Autodesk Inventor part; units mm, degrees
ref_plane "YZ Plane" through (0, 0, 0) normal (1, 0, 0) x (0, 1, 0)
ref_plane "XZ Plane" through (0, 0, 0) normal (0, 1, 0) x (-1, 0, 0)
ref_plane "XY Plane" through (0, 0, 0) normal (0, 0, 1) x (1, 0, 0)
sketch "Skizze1" plane through (0, 0, 0) normal (1, 0, 0) x (0, 1, 0)
  line L0 (-35, 0) -> (35, 0) construction
  line L1 (0, 42) -> (0, -42) construction
  line L2 (-25, -30) -> (25, -30)
  line L3 (25, -30) -> (25, 30)
  line L4 (25, 30) -> (-25, 30)
  line L5 (-25, 30) -> (-25, -30)
  line L6 (-25, -30) -> (25, 30) construction
  line L7 (25, -30) -> (-25, 30) construction
  point P0 (0, 0)
  dimension "d0" = 50
  dimension "d1" = 60
extrude "Grundkörper" add sketch "Skizze1" along normal mid plane 30
sketch "Skizze2" plane through (15, 0, 0) normal (1, 0, 0) x (0, 0, -1)
  line L0 (-30, 25) -> (-30, -25) construction
  line L1 (0, -35) -> (0, 35) construction
  line L2 (-42, 0) -> (42, 0) construction
  line L3 (-30, -15) -> (10, -15)
  line L4 (10, -15) -> (10, 15)
  line L5 (10, 15) -> (-30, 15)
  line L6 (-30, 15) -> (-30, -15)
  line L7 (30, -25) -> (30, 25) construction
  line L8 (30, -8.4) -> (25, -8.4)
  line L9 (17, -0.4) -> (17, 0.4)
  line L10 (25, 8.4) -> (30, 8.4)
  line L11 (30, -8.4) -> (30, 8.4)
  arc A0 (17, -0.4) -> (25, -8.4) centre (25, -0.4) ccw
  arc A1 (25, 8.4) -> (17, 0.4) centre (25, 0.4) ccw
  point P0 (0, 0)
  dimension "d4" = 40
  dimension "d5" = 30
  dimension "d14" = 13
  dimension "d15" = 16.8
  dimension "d16" = 8
extrude "Ausschnitt" cut sketch "Skizze2" against normal through all
sketch "Skizze4" plane through (-15, -25, -30) normal (0, -1, 0) x (1, 0, 0)
  line L0 (30, 20) -> (0, 20) construction
  line L1 (30, 60) -> (0, 60) construction
  line L2 (15, 72) -> (15, -12)
  line L3 (0, 40) -> (30, 40) construction
  line L4 (0, 0) -> (0, 60) construction
  line L5 (30, 60) -> (30, 0) construction
  point P0 (15, 30)
  point P1 (15, 50)
  point P2 (15, 30)
  dimension "d19" = 40
  dimension "d20" = 20
  dimension "d21" = 20
hole "DIN7984_M8_Boh" at (0, -25, 20) at (0, -25, 0) direction (0, 1, 0) diameter 9 end up to surface counterbore diameter 15 counterbore depth 5.4
mirror "Spiegeln_DIN7984_M8_Boh" about plane through (0, 0, 0) normal (0, 1, 0) of "DIN7984_M8_Boh"
sketch "Skizze5" plane through (15, -25, -30) normal (0, 0, -1) x (-1, 0, 0)
  line L0 (0, 0) -> (30, 0) construction
  line L1 (30, 16.6) -> (0, 16.6) construction
  line L2 (30, 50) -> (0, 50) construction
  line L3 (0, 33.4) -> (30, 33.4) construction
  line L4 (15, -10) -> (15, 60) construction
  line L5 (-6, 25) -> (36, 25) construction
  line L6 (15, 16.6) -> (15, 0) construction
  point P0 (15, 25)
  point P1 (15, 8.3)
  point P2 (15, 41.7)
  dimension "d29" = 33.4
hole "M5x10" at (0, -16.7, -30) at (0, 16.7, -30) direction (0, 0, 1) diameter 4.134 depth 14.2 tip angle 118 countersink diameter 5 countersink angle 90
sketch "Skizze" plane through (15, -25, -30) normal (0, 0, -1) x (-1, 0, 0)
  circle A0 centre (15, 8.3) radius 2.5
  line L0 (30, 16.6) -> (0, 16.6)
  line L1 (0, 0) -> (0, 16.6)
  line L2 (0, 0) -> (30, 0)
  line L3 (30, 16.6) -> (30, 0)
  circle A1 centre (15, 41.7) radius 2.5
  line L4 (0, 33.4) -> (30, 33.4)
  line L5 (30, 50) -> (30, 33.4)
  line L6 (30, 50) -> (0, 50)
  line L7 (0, 33.4) -> (0, 50)
  line L8 (0, 16.6) -> (0, 24.6)
  line L9 (0, 24.6) -> (0, 25.4)
  line L10 (0, 25.4) -> (0, 33.4)
  line L11 (30, 33.4) -> (30, 25.4)
  line L12 (30, 25.4) -> (30, 24.6)
  line L13 (30, 24.6) -> (30, 16.6)
  point P0 (15, 25)
chamfer "Fase_Allgemein" distance 4 angle 45 4 edges at (15, -25, 0) (-15, -25, 0) (15, 25, 0) (-15, 25, 0)
chamfer "Fase" distance 0.5 angle 45 15 edges at (15, -6.0569, -19.3431) (15, 0, -17) (15, 6.0569, -19.3431) (15, 8.4, -27.5) (15, -8.4, -27.5) (-15, 6.0569, -19.3431) (-15, 0, -17) (-15, -6.0569, -19.3431) (-15, -8.4, -27.5) (-15, 8.4, -27.5) (-15, 0, -10) (-15, 15, 10) (15, -15, 10) (15, 0, -10) (15, 15, 10)
equation "\"d20\" = 0.5 * d19"
properties part number "200-50-WHEEL-CONNECTOR-30MM-01" material "Aluminium 6061"
The listing builds one solid part. Answer for the finished solid, in the listing's coordinates (mm). A direction names the side the tool comes from. Round coordinates to 2 decimals unless told otherwise and drop trailing zeros. Order: outer loops, then holes, each group sorted by start corner. A loop starts at its lowest first (then second) coordinate and runs counter-clockwise, first axis right, second up. Notation, with made-up numbers: (22, 59) -> (36, 59) arc R18 cw to (36, 67) -> close; hole circle Ø4 at (15, 84.25). An arc over 180 degrees is marked (long way). Answer as CSV lines item,"result". Start each with the question number.
(1) A tool of negligible diameter and unlimited length cuts with its end or side. For faces 5 (the face through (0, 19.6, 25)), 6 (the face through (0, -19.6, 15)), 7 (the face through (0.203, 6.119, -19.406)), 8 (the face through (0, -15, 10)), from which of +Z, -Z, +X, -X, +Y, -Y can it reach the whole face along a straight path? Write none if from no direction.
(2) Flat-ended cylindrical pins translate along their axes: pin 1 Ø11.5 at (x, z) = (0, 0) entering from +Y; pin 2 Ø9 at (x, z) = (-6, 3.5) entering from +Y; pin 3 Ø2 at (x, y) = (-0.5, 13.5) entering from +Z; pin 4 Ø0.9 at (x, y) = (-7, 0) entering from -Z. Find the tip coordinate at first contact, or state that the pin passes through.
(3) For a pull along X with two mould halves and no side action, classify faces 1 (the face through (14.64, 6.22, -19.31)), 2 (the face through (-4.46, -17.27, 0.59)), 3 (the face through (-13, -23, 0)), 4 (the face through (0, -20, 30)) as +X half, -X half, draft (parallel to the pull), parting line (faces both ways), or undercut.
(4) The part is cut by section C-C (x = -10). Determine the outline of the cut face in (y, z).
(5) Find the intervals of material crossed by probe 1 along Y at (x, z) = (0, -27); probe 2 along Y at (x, z) = (-2, 5.5); probe 3 along Z at (x, y) = (0, 21), in increasing order. Write a range as from..to.
(6) The part is cut by section A-A (z = 20). Count the separate pieces of the cut face and the enclosed holes in it, then the cut area to 3 significant figures.
(7) The part is cut by section B-B (z = 10.5). Determine the outline of the cut face in (x, y), then the cut area to 3 significant figures.
Evaluation:
1,face 5,"+Y"
1,face 6,"-Y"
1,face 7,"-Z, +X, -X"
1,face 8,"+Z, +X, -X"
2,pin 1,"y = 19.6"
2,pin 2,"y = 25"
2,pin 3,"z = -10"
2,pin 4,"z = -17"
3,face 1,"+X half"
3,face 2,"undercut"
3,face 3,"-X half"
3,face 4,"draft"
4,outline,"(-25, -30) -> (-8.4, -30) -> (-8.4, -25) arc R8 cw to (-0.4, -17) -> (0.4, -17) arc R8 cw to (8.4, -25) -> (8.4, -30) -> (25, -30) -> (25, 30) -> (15, 30) -> (15, -10) -> (-15, -10) -> (-15, 30) -> (-25, 30) -> close"
5,probe 1,"-25..-18.77, -14.63..-8.4, 8.4..14.63, 18.77..25"
5,probe 2,"-19.6..-15, 15..19.6"
5,probe 3,"-30..-7.5, 7.5..12.5, 27.5..30"
6,separate pieces,"4"
6,enclosed holes,"0"
6,area,"323 mm²"
7,outline,"(-15, -21) -> (-11, -25) -> (11, -25) -> (15, -21) -> (15, -15.5) -> (14.5, -15) -> (-15, -15) -> close; (-15, 15.5) -> (-14.5, 15) -> (14.5, 15) -> (15, 15.5) -> (15, 21) -> (11, 25) -> (-11, 25) -> (-15, 21) -> close"
7,area,"568 mm²"
